Model file for the job. Use its own axes, mm. Give positions to 0.01 mm unless a question says otherwise; leave off trailing zeros. Write each loop counter-clockwise with the first axis right and the second up, starting at its lowest first coordinate (ties: lowest second). Pieces come first, ordered by that corner, then holes. Notation, with made-up numbers: (-36, -13.5) - (15, -13.5) arc R10 cw to (15, 1.5) - close; hole circle Ø7 at (57.5, 66). An arc over 180 degrees is marked (long way). Use a Markdown table: item, result. Add a question column.
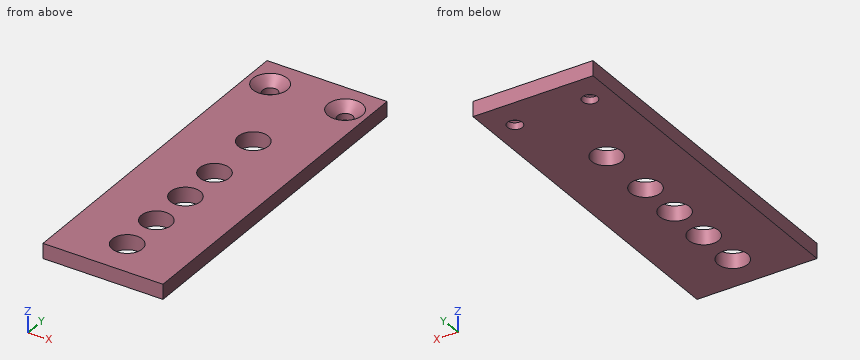
```python
from build123d import *

# Parameters (mm, degrees)
SKETCH1_W           = 50.8
SKETCH1_H           = 146.685
SKETCH1_R           = 6.35
SKETCH1_R_2         = 3.175
BOSS_EXTRUDE3_DEPTH = 6.35
CHAMFER1_SIZE       = 4.0894
CHAMFER1_SIZE2      = 3.554861186
CHAMFER2_SIZE       = 4.0894
CHAMFER2_SIZE2      = 3.554861186


with BuildPart() as part:
    # Sketch1 → Boss-Extrude3 (new body)
    with BuildSketch(Plane.XY):
        with Locations((0, -73.3425)):
            Rectangle(SKETCH1_W, SKETCH1_H)
        with Locations((0, -130.81)):
            Circle(SKETCH1_R, mode=Mode.SUBTRACT)
        with Locations((0, -111.76)):
            Circle(SKETCH1_R, mode=Mode.SUBTRACT)
        with Locations((0, -92.71)):
            Circle(SKETCH1_R, mode=Mode.SUBTRACT)
        with Locations((0, -73.66)):
            Circle(SKETCH1_R, mode=Mode.SUBTRACT)
        with Locations((-15.875, -12.7)):
            Circle(SKETCH1_R_2, mode=Mode.SUBTRACT)
        with Locations((15.875, -12.7)):
            Circle(SKETCH1_R_2, mode=Mode.SUBTRACT)
        with Locations((0, -48.26)):
            Circle(SKETCH1_R, mode=Mode.SUBTRACT)
    extrude(amount=BOSS_EXTRUDE3_DEPTH)

    # Chamfer1
    chamfer1_edges = [part.edges().sort_by_distance(p)[0] for p in [
        (-19.05, -12.7, 6.35),
    ]]
    chamfer1_side = [part.faces().sort_by_distance(p)[0] for p in [
        (0, -145.132674995, 6.35),
    ]]
    chamfer(chamfer1_edges, length=CHAMFER1_SIZE, length2=CHAMFER1_SIZE2, reference=chamfer1_side[0])

    # Chamfer2
    chamfer2_edges = [part.edges().sort_by_distance(p)[0] for p in [
        (12.7, -12.7, 6.35),
    ]]
    chamfer2_side = [part.faces().sort_by_distance(p)[0] for p in [
        (-24.691725005, -12.7, 6.35),
    ]]
    chamfer(chamfer2_edges, length=CHAMFER2_SIZE, length2=CHAMFER2_SIZE2, reference=chamfer2_side[0])


solid = part.part
```
(1) Probe probe 1 along Y at (x, z) = (0, 6.25) (3 decimals); probe 2 along Y at (x, z) = (0.5, 4.5) (3 decimals); probe 3 along X at (y, z) = (-10.5, 4). List the from-to ranges inside material, lowest first. Write a range as [from, to].
(2) Band-saw the part on C-C (z = 1.75). Write the cut outline in (x, y) (3 decimals), then the cut area to 3 significant figures.
(3) Band-saw the part on A-A (y = -48.26). Write the cut outline in (x, z).
(4) Band-saw the part on D-D (y = -70). Write the cut outline in (x, z).
(5) Band-saw the part on B-B (x = 0). Write the cut outline in (y, z) (3 decimals), then the cut area to 3 significant figures.
Model answer:
| question | item | result |
|---|---|---|
| 1 | probe 1 | y = [-146.685, -137.16], [-124.46, -118.11], [-105.41, -99.06], [-86.36, -80.01], [-67.31, -54.61], [-41.91, 0] |
| 1 | probe 2 | y = [-146.685, -137.14], [-124.48, -118.09], [-105.43, -99.04], [-86.38, -79.99], [-67.33, -54.59], [-41.93, 0] |
| 1 | probe 3 | x = [-25.4, -19.87], [-11.88, 11.88], [19.87, 25.4] |
| 2 | outline | (-25.4, -146.685) - (25.4, -146.685) - (25.4, 0) - (-25.4, 0) - close; hole circle Ø6.35 at (-15.875, -12.7); hole circle Ø12.7 at (0, -130.81); hole circle Ø12.7 at (0, -111.76); hole circle Ø12.7 at (0, -92.71); hole circle Ø12.7 at (0, -73.66); hole circle Ø12.7 at (0, -48.26); hole circle Ø6.35 at (15.875, -12.7) |
| 2 | area | 6,750 mm^2 |
| 3 | outline | (-25.4, 0) - (-6.35, 0) - (-6.35, 6.35) - (-25.4, 6.35) - close; (6.35, 0) - (25.4, 0) - (25.4, 6.35) - (6.35, 6.35) - close |
| 4 | outline | (-25.4, 0) - (-5.19, 0) - (-5.19, 6.35) - (-25.4, 6.35) - close; (5.19, 0) - (25.4, 0) - (25.4, 6.35) - (5.19, 6.35) - close |
| 5 | outline | (-146.685, 0) - (-137.16, 0) - (-137.16, 6.35) - (-146.685, 6.35) - close; (-124.46, 0) - (-118.11, 0) - (-118.11, 6.35) - (-124.46, 6.35) - close; (-105.41, 0) - (-99.06, 0) - (-99.06, 6.35) - (-105.41, 6.35) - close; (-86.36, 0) - (-80.01, 0) - (-80.01, 6.35) - (-86.36, 6.35) - close; (-67.31, 0) - (-54.61, 0) - (-54.61, 6.35) - (-67.31, 6.35) - close; (-41.91, 0) - (0, 0) - (0, 6.35) - (-41.91, 6.35) - close |
| 5 | area | 528 mm^2 |
